Read the model definition and answer for the solid it produces. Units are mm, in the model's axes. A direction names the side the tool comes from. Give positions to 0.01 mm unless a question says otherwise; leave off trailing zeros. Order: outer loops, then holes, each group sorted by start corner. A loop starts at its lowest first (then second) coordinate and runs counter-clockwise, first axis right, second up. Notation, with made-up numbers: (37, 56) - (42, 56) arc R29 ccw to (42, 95) - close; hole circle Ø9 at (-13.5, 50). An arc over 180 degrees is marked (long way). Write each question's results on one line, items separated by ' | '. Start each with the question number.
Q1. For a pull along Y with two mould halves and no side action, classify faces 1 (the face through (-65, 10, 0)), 2 (the face through (-53.57, -41.07, 2.46)), 3 (the face through (-5.598, 42.634, 8.986)) as +Y half, -Y half, draft (parallel to the pull), parting line (faces both ways), or undercut.
Q2. Find the intervals of material crossed by line 1 along Y through (x, z) = (0, 9); line 2 along Y through (x, z) = (0, 8.8); line 3 along Z through (x, y) = (-54.5, -15), in increasing order. Write a range as from..to.
Q3. Find section C-C on z = 1.5. Give the vertices of the cut face in (x, y).
Q4. Find section A-A on x = 0. Give the vertices of the cut face in (y, z), and give its area (3 significant figures).
Q5. A tool of negligible diameter and unlimited length cuts with its end or side. For faces 4 (the face through (-15, -41, 10)), 5 (the face through (62.475, 19.674, 1.479)), from which of +Z, -Z, +X, -X, +Y, -Y can it reach the whole face along a straight path? Write none if from no direction.
Q6. Flat-ended cylindrical pins translate along their axes: P1, Ø1.5, axis at x = -34.5, z = 8.5, coming from the +Y side; P2, Ø5, axis at y = 39.5, z = 7.5, coming from the +X side; P3, Ø5, axis at y = 8.5, z = 3, coming from the -X side. Find the tip coordinate at first contact, or state that the pin passes through.
from build123d import *

# Parameters (mm, degrees)
F0_R     = 67.5
F0_R_2   = 65.5
F0_R_3   = 43
F1_DEPTH = 10
F2_DEPTH = 8
F3_R     = 5


with BuildPart() as f1:
    # F0 (on Top) → F1 (new body)
    with BuildSketch(Plane.XY):
        Circle(F0_R)
        Circle(F0_R_2, mode=Mode.SUBTRACT)
        Circle(F0_R_2)
        Circle(F0_R_3, mode=Mode.SUBTRACT)
    extrude(amount=F1_DEPTH)

    # F0 (on Top) → F2 (cut)
    with BuildSketch(Plane.XY):
        Circle(F0_R_2)
        Circle(F0_R_3, mode=Mode.SUBTRACT)
    extrude(amount=F2_DEPTH, mode=Mode.SUBTRACT)

    # F3
    f3_edges = [f1.edges().sort_by_distance(p)[0] for p in [
        (-65.5, 0, 8),
        (-67.5, 0, 10),
    ]]
    fillet(f3_edges, radius=F3_R)


solid = f1.part
Working result:
1) face 1: draft | face 2: parting line | face 3: undercut
2) line 1: -65.5..-43, 43..65.5 | line 2: -65.75..-43, 43..65.75 | line 3: 8..10
3) outline: circle Ø135 at (0, 0); hole circle Ø131 at (0, 0)
4) outline: (-67.5, 0) - (-65.5, 0) - (-65.5, 3) arc R5 cw to (-60.5, 8) - (-43, 8) - (-43, 10) - (-62.5, 10) arc R5 ccw to (-67.5, 5) - close; (43, 8) - (60.5, 8) arc R5 cw to (65.5, 3) - (65.5, 0) - (67.5, 0) - (67.5, 5) arc R5 ccw to (62.5, 10) - (43, 10) - close | area: 130 mm²
5) face 4: +Z, +X, -X, +Y, -Y | face 5: -Z
6) P1: y = 57.21 | P2: x = 56.05 | P3: x = -67.23
